Autodesk Inventor part; units mm, degrees
ref_plane "YZ Plane" through (0, 0, 0) normal (1, 0, 0) x (0, 1, 0)
ref_plane "XZ Plane" through (0, 0, 0) normal (0, 1, 0) x (-1, 0, 0)
ref_plane "XY Plane" through (0, 0, 0) normal (0, 0, 1) x (1, 0, 0)
sketch "Sketch1" plane through (0, 0, 0) normal (0, 1, 0) x (-1, 0, 0)
  circle A0 centre (0, 0) radius 10.5
  line L0 (0, 0) -> (0, -23.5)
  circle A1 centre (0, -23.5) radius 5.25
  line L1 (0, -23.5) -> (0, -35.25)
  line L2 (-14, -35.25) -> (-14, -58.75)
  line L3 (-14, -58.75) -> (-19, -58.75)
  line L4 (-19, -58.75) -> (-19, -35.25)
  line L5 (-35.25, 21.625) -> (35.25, 21.625)
  line L6 (-35.25, 21.625) -> (35.25, 21.625) construction
  line L7 (35.25, 21.625) -> (25.25, 21.625)
  line L8 (-35.25, 21.625) -> (35.25, 21.625)
  line L9 (35.25, 21.625) -> (35.25, -69.875)
  line L10 (35.25, -69.875) -> (-35.25, -69.875)
  line L11 (-35.25, 11.625) -> (-35.25, 21.625)
  line L12 (-35.25, 21.625) -> (-35.25, 11.625)
  line L13 (-35.25, 11.625) -> (-25.25, 11.625)
  circle A2 centre (-25.25, 11.625) radius 3.5
  line L14 (35.25, 21.625) -> (25.25, 21.625)
  line L15 (25.25, 21.625) -> (25.25, 11.625)
  circle A3 centre (25.25, 11.625) radius 3.5
  line L16 (35.25, -69.875) -> (25.25, -69.875)
  line L17 (25.25, -69.875) -> (25.25, -59.875)
  circle A4 centre (25.25, -59.875) radius 3.5
  line L18 (-35.25, -69.875) -> (-25.25, -69.875)
  line L19 (-25.25, -69.875) -> (-25.25, -59.875)
  circle A5 centre (-25.25, -59.875) radius 3.5
  line L20 (-25.25, 11.625) -> (-25.25, -18.375)
  line L21 (25.25, -59.875) -> (25.25, -29.875)
  circle A6 centre (-25.25, -18.375) radius 2.5
  circle A7 centre (25.25, -29.875) radius 2.5
  line L22 (-19, -35.25) -> (-14, -35.25)
  line L23 (35.25, -69.875) -> (15.25, -69.875)
  line L24 (15.25, -69.875) -> (15.25, 21.625)
  dimension "d0" = 21
  dimension "d1" = 23.5
  dimension "d2" = 10.5
  dimension "d3" = 11.75
  dimension "d5" = 23.5
  dimension "d6" = 5
  dimension "d7" = 23.5
  dimension "d9" = 70.5
  dimension "d40" = 21.625
  dimension "d41" = 70.5
  dimension "d42" = 91.5
  dimension "d43" = 10
  dimension "d44" = 10
  dimension "d45" = 7
  dimension "d46" = 10
  dimension "d47" = 10
  dimension "d48" = 90
  dimension "d50" = 7
  dimension "d51" = 10
  dimension "d52" = 10
  dimension "d53" = 7
  dimension "d54" = 10
  dimension "d55" = 10
  dimension "d56" = 7
  dimension "d60" = 30
  dimension "d61" = 30
  dimension "d62" = 5
  dimension "d63" = 5
  dimension "d64" = 14
  dimension "d65" = 20
extrude "Extrusion1" add sketch "Sketch1" along normal blind 4 contours L5 L9 L10 L24
properties part number "m"
The listing builds one solid part. Answer for the finished solid, in the listing's coordinates (mm). Give positions to 0.01 mm unless a question says otherwise; leave off trailing zeros. Write each loop counter-clockwise with the first axis right and the second up, starting at its lowest first coordinate (ties: lowest second). Pieces come first, ordered by that corner, then holes. Notation, with made-up numbers: (87.25, 77.25) -> (91.25, 77.25) arc R10 cw to (91.25, 93.25) -> close; hole circle Ø5 at (44.25, -15.75). An arc over 180 degrees is marked (long way). One line per question, with ' | ' between items. Start each with the question number.
1. Section B-B (y = 0.9) is taken. Determine the outline of the cut face in (x, z) (3 decimals), plus the area to 3 significant figures.
2. Find the intervals of material crossed by probe 1 along Z at (x, y) = (-25.25, 2.55) (3 decimals); probe 2 along Z at (x, y) = (-27, 1.5) (3 decimals); probe 3 along X at (y, z) = (0.5, -30), in increasing order.
3. For a pull along Z with two mould halves and no side action, classify faces 1 (the flat face through (-25, 2, -69.875)), 2 (the flat face through (-25, 4, -23)), 3 (the cylindrical face through (-28.588, 1.972, -60.926)) as pulls with the +Z half, pulls with the -Z half, needs draft (parallel to the pull), parting line crosses it, or undercut.
4. Section A-A (x = -25.25) is taken. Determine the outline of the cut face in (y, z) (3 decimals), plus the area to 3 significant figures.
Response values:
1) outline: (-35.25, -69.875) -> (-15.25, -69.875) -> (-15.25, 21.625) -> (-35.25, 21.625) -> close; hole circle Ø7 at (-25.25, -59.875); hole circle Ø7 at (-25.25, 11.625); hole circle Ø5 at (-25.25, -29.875) | area: 1,730 mm2
2) probe 1: -69.875 to -63.375, -56.375 to -32.375, -27.375 to 8.125, 15.125 to 21.625 | probe 2: -69.875 to -62.906, -56.844 to -31.66, -28.09 to 8.594, 14.656 to 21.625 | probe 3: -35.25 to -27.75, -22.75 to -15.25
3) face 1: pulls with the -Z half | face 2: needs draft | face 3: undercut
4) outline: (0, -69.875) -> (4, -69.875) -> (4, -63.375) -> (0, -63.375) -> close; (0, -56.375) -> (4, -56.375) -> (4, -32.375) -> (0, -32.375) -> close; (0, -27.375) -> (4, -27.375) -> (4, 8.125) -> (0, 8.125) -> close; (0, 15.125) -> (4, 15.125) -> (4, 21.625) -> (0, 21.625) -> close | area: 290 mm2
